Check sheet for the modelled part. Datum: model origin and axes. Units: mm. A direction names the side the tool comes from. Give positions to 0.01 mm unless a question says otherwise; leave off trailing zeros. Order: outer loops, then holes, each group sorted by start corner. A loop starts at its lowest first (then second) coordinate and runs counter-clockwise, first axis right, second up. Notation, with made-up numbers: (29.25, -3.75) - (58.25, -3.75) arc R25 ccw to (58.25, 20.25) - close; hole circle Ø7 at (-28.75, 39). An arc over 180 degrees is marked (long way). Answer in a Markdown table with one row per item.
from build123d import *

# Parameters (mm, degrees)
SALIENTE_EXTRUIR1_DEPTH = 10
CROQUIS2_W              = 10
CROQUIS2_H              = 5
SALIENTE_EXTRUIR2_DEPTH = 10
CROQUIS4_R              = 1.5
CORTAR_EXTRUIR1_DEPTH   = 10
CROQUIS5_R              = 1.5
CORTAR_EXTRUIR2_DEPTH   = 9.5
SKETCH1_W               = 10
SKETCH1_H               = 2.5
CUT_EXTRUDE1_DEPTH      = 10


with BuildPart() as part:
    # Croquis1 → Saliente-Extruir1 (new body)
    with BuildSketch(Plane(origin=(0, 0, 0), x_dir=(1, 0, 0), z_dir=(0, 1, 0))):
        Polygon((-50, 2.5), (-50, 5), (50, 5), (50, -5), (-50, -5), (-50, -2.5), (-35, -2.5), (-35, 2.5), align=None)
    extrude(amount=SALIENTE_EXTRUIR1_DEPTH)

    # Croquis2 → Saliente-Extruir2 (add)
    with BuildSketch(Plane(origin=(50, 0, 0), x_dir=(0, 0, -1), z_dir=(1, 0, 0))):
        with Locations((0, 5)):
            Rectangle(CROQUIS2_W, CROQUIS2_H)
    extrude(amount=SALIENTE_EXTRUIR2_DEPTH)

    # Croquis4 → Cortar-Extruir1 (cut)
    with BuildSketch(Plane(origin=(0, 7.5, 0), x_dir=(1, 0, 0), z_dir=(0, 1, 0))):
        with Locations(Location((55, 0, 0), (0, 0, 270))):
            Circle(CROQUIS4_R)
        with BuildLine():
            Line((55, 5), (55, 11.029230351))
            Line((55, 11.029230351), (66.142651686, 11.029230351))
            Line((66.142651686, 11.029230351), (66.142651686, -12.901676623))
            Line((66.142651686, -12.901676623), (58.757445268, -12.901676623))
            Line((58.757445268, -12.901676623), (55, -5))
            ThreePointArc((55, -5), (60, 0), (55, 5))
        make_face()
    extrude(amount=-CORTAR_EXTRUIR1_DEPTH, mode=Mode.SUBTRACT)

    # Croquis5 → Cortar-Extruir2 (cut, symmetric)
    with BuildSketch(Plane(origin=(0, 0, 2.5), x_dir=(-1, 0, 0), z_dir=(0, 0, -1))):
        with Locations((45, 5)):
            Circle(CROQUIS5_R)
    extrude(amount=CORTAR_EXTRUIR2_DEPTH, both=True, mode=Mode.SUBTRACT)

    # Sketch1 → Cut-Extrude1 (cut)
    with BuildSketch(Plane(origin=(50, 0, 0), x_dir=(0, 0, -1), z_dir=(1, 0, 0))):
        with Locations((0, 8.75)):
            Rectangle(SKETCH1_W, SKETCH1_H)
        with Locations((0, 1.25)):
            Rectangle(SKETCH1_W, SKETCH1_H)
    extrude(amount=-CUT_EXTRUDE1_DEPTH, mode=Mode.SUBTRACT)


solid = part.part
(1) Thickness scan on L1, parallel to Y at x = -45, z = -4.3; L2, parallel to Z at x = -39, y = 1.75; L3, parallel to X at y = 8.5, z = 4.25. Record the ranges inside material, lowest first.
Geometry says:
| item | result |
|---|---|
| L1 | 0 to 3.5, 6.5 to 10 |
| L2 | -5 to -2.5, 2.5 to 5 |
| L3 | -50 to 40 |
(2) Mould release check, pull along X, two halves, no side actions. Record for faces 1 (the cylindrical face through (56.01, 5.04, -1.11)), 2 (the flat face through (2, 5, -5)), 3 (the flat face through (-50, 5, -4)): pulls with the +X half, pulls with the -X half, needs draft (parallel to the pull), parting line crosses it, or undercut.
Geometry says:
| item | result |
|---|---|
| face 1 | undercut |
| face 2 | needs draft |
| face 3 | pulls with the -X half |
(3) Gauge pin test, flat ends, axial feed: P1, Ø0.8, axis at y = 1.5, z = 1, coming from the +X side; P2, Ø2, axis at y = 6.5, z = 1.5, coming from the +X side; P3, Ø5, axis at x = 55, z = 0, coming from the +Y side. Record the tip position at first contact, or that the pin passes through.
Geometry says:
| item | result |
|---|---|
| P1 | x = 40 |
| P2 | x = 59.97 |
| P3 | y = 7.5 |
(4) Cross-section at D-D, the plane x = 43.5. Record the cut outline in (y, z).
Geometry says:
| item | result |
|---|---|
| outline | (2.5, -5) - (7.5, -5) - (7.5, 5) - (2.5, 5) - close |
(5) Access from +Z, -Z, +X, -X, +Y, -Y to the whole of each face (thin tool, end or side, straight path). Record for faces 4 (the cylindrical face through (-43.5, 5.07, -3.77)), 5 (the flat face through (-35, 5, 0)), 6 (the flat face through (50, 7.5, 0)), 7 (the flat face through (40, 1, 0)).
Geometry says:
| item | result |
|---|---|
| face 4 | +Z, -Z |
| face 5 | -X, +Y, -Y |
| face 6 | +Z, -Z, +X, +Y |
| face 7 | +Z, -Z, +X, -Y |
(6) Cross-section at A-A, the plane z = 0. Record the cut outline in (x, y), then the cut area to 3 significant figures.
Geometry says:
| item | result |
|---|---|
| outline | (-35, 0) - (40, 0) - (40, 2.5) - (53.5, 2.5) - (53.5, 7.5) - (40, 7.5) - (40, 10) - (-35, 10) - close; (56.5, 2.5) - (60, 2.5) - (60, 7.5) - (56.5, 7.5) - close |
| area | 835 mm² |
(7) Cross-section at C-C, the plane y = 8.75. Record the cut outline in (x, z).
Geometry says:
| item | result |
|---|---|
| outline | (-50, -5) - (40, -5) - (40, 5) - (-50, 5) - (-50, 2.5) - (-35, 2.5) - (-35, -2.5) - (-50, -2.5) - close |
(8) Cross-section at B-B, the plane x = -45. Record the cut outline in (y, z).
Geometry says:
| item | result |
|---|---|
| outline | (0, -5) - (3.5, -5) - (3.5, -2.5) - (0, -2.5) - close; (0, 2.5) - (3.5, 2.5) - (3.5, 5) - (0, 5) - close; (6.5, -5) - (10, -5) - (10, -2.5) - (6.5, -2.5) - close; (6.5, 2.5) - (10, 2.5) - (10, 5) - (6.5, 5) - close |
